from build123d import *

# Parameters (mm, degrees)
ESBO_O1_W                = 111
ESBO_O1_H                = 40
RESSALTO_EXTRUS_O1_DEPTH = 18
ESBO_O2_W                = 2
ESBO_O2_H                = 16
ESBO_O2_H_2              = 21
ESBO_O2_H_3              = 40
RESSALTO_EXTRUS_O2_DEPTH = 13
RESSALTO_EXTRUS_O3_REACH = 68.643
ESBO_O3_W                = 3
ESBO_O3_H                = 7.5
ESBO_O4_R                = 1.65
CORTE_EXTRUS_O1_DEPTH    = 6
FILETE1_R                = 5


with BuildPart() as part:
    # Esboço1 → Ressalto-extrusão1 (new body)
    with BuildSketch(Plane.XY):
        Rectangle(ESBO_O1_W, ESBO_O1_H)
    extrude(amount=RESSALTO_EXTRUS_O1_DEPTH)

    # Esboço2 → Ressalto-extrusão2 (add)
    with BuildSketch(Plane.XY.offset(18)):
        with Locations((-28.2, -12)):
            Rectangle(ESBO_O2_W, ESBO_O2_H)
        with Locations((-23.072727273, -12)):
            Rectangle(ESBO_O2_W, ESBO_O2_H)
        with Locations((-17.945454545, -12)):
            Rectangle(ESBO_O2_W, ESBO_O2_H)
        with Locations((-12.818181818, -12)):
            Rectangle(ESBO_O2_W, ESBO_O2_H)
        with Locations((-7.690909091, -12)):
            Rectangle(ESBO_O2_W, ESBO_O2_H)
        with Locations((-2.563636364, -12)):
            Rectangle(ESBO_O2_W, ESBO_O2_H)
        with Locations((2.563636364, -12)):
            Rectangle(ESBO_O2_W, ESBO_O2_H)
        with Locations((7.690909091, -12)):
            Rectangle(ESBO_O2_W, ESBO_O2_H)
        with Locations((12.818181818, -12)):
            Rectangle(ESBO_O2_W, ESBO_O2_H)
        with Locations((17.945454545, -12)):
            Rectangle(ESBO_O2_W, ESBO_O2_H)
        with Locations((23.072727273, -12)):
            Rectangle(ESBO_O2_W, ESBO_O2_H)
        with Locations((28.2, -12)):
            Rectangle(ESBO_O2_W, ESBO_O2_H)
        with Locations((-47.9, 0)):
            Rectangle(ESBO_O2_W, ESBO_O2_H_2)
        with Locations((-52.9, 0)):
            Rectangle(ESBO_O2_W, ESBO_O2_H_2)
        with Locations((-42.9, 0)):
            Rectangle(ESBO_O2_W, ESBO_O2_H_3)
        with Locations((-37.9, 0)):
            Rectangle(ESBO_O2_W, ESBO_O2_H_3)
        with Locations((-32.9, 0)):
            Rectangle(ESBO_O2_W, ESBO_O2_H_3)
        with Locations((32.9, 0)):
            Rectangle(ESBO_O2_W, ESBO_O2_H_3)
        with Locations((37.9, 0)):
            Rectangle(ESBO_O2_W, ESBO_O2_H_3)
        with Locations((42.9, 0)):
            Rectangle(ESBO_O2_W, ESBO_O2_H_3)
        with Locations((47.9, 0)):
            Rectangle(ESBO_O2_W, ESBO_O2_H_2)
        with Locations((52.9, 0)):
            Rectangle(ESBO_O2_W, ESBO_O2_H_2)
    extrude(amount=RESSALTO_EXTRUS_O2_DEPTH)

    # Esboço3 → Ressalto-extrusão3 (add, up to next)
    with BuildSketch(Plane.XY.offset(31), mode=Mode.PRIVATE) as ressalto_extrus_o3_sk1:
        with Locations((-40.4, -11.95)):
            Rectangle(ESBO_O3_W, ESBO_O3_H)
    ressalto_extrus_o3_tool1 = extrude(ressalto_extrus_o3_sk1.sketch, amount=-RESSALTO_EXTRUS_O3_REACH, mode=Mode.PRIVATE) - part.part
    # Esboço3 → Ressalto-extrusão3 (add, up to next)
    with BuildSketch(Plane.XY.offset(31), mode=Mode.PRIVATE) as ressalto_extrus_o3_sk2:
        with Locations((-35.4, -11.95)):
            Rectangle(ESBO_O3_W, ESBO_O3_H)
    ressalto_extrus_o3_tool2 = extrude(ressalto_extrus_o3_sk2.sketch, amount=-RESSALTO_EXTRUS_O3_REACH, mode=Mode.PRIVATE) - part.part
    # Esboço3 → Ressalto-extrusão3 (add, up to next)
    with BuildSketch(Plane.XY.offset(31), mode=Mode.PRIVATE) as ressalto_extrus_o3_sk3:
        with Locations((35.4, -11.95)):
            Rectangle(ESBO_O3_W, ESBO_O3_H)
    ressalto_extrus_o3_tool3 = extrude(ressalto_extrus_o3_sk3.sketch, amount=-RESSALTO_EXTRUS_O3_REACH, mode=Mode.PRIVATE) - part.part
    # Esboço3 → Ressalto-extrusão3 (add, up to next)
    with BuildSketch(Plane.XY.offset(31), mode=Mode.PRIVATE) as ressalto_extrus_o3_sk4:
        with Locations((40.4, -11.95)):
            Rectangle(ESBO_O3_W, ESBO_O3_H)
    ressalto_extrus_o3_tool4 = extrude(ressalto_extrus_o3_sk4.sketch, amount=-RESSALTO_EXTRUS_O3_REACH, mode=Mode.PRIVATE) - part.part
    add(ressalto_extrus_o3_tool1.solids().sort_by_distance((-40.4, -11.95, 31))[0])
    add(ressalto_extrus_o3_tool2.solids().sort_by_distance((-35.4, -11.95, 31))[0])
    add(ressalto_extrus_o3_tool3.solids().sort_by_distance((35.4, -11.95, 31))[0])
    add(ressalto_extrus_o3_tool4.solids().sort_by_distance((40.4, -11.95, 31))[0])

    # Esboço4 → Corte-extrusão1 (cut)
    with BuildSketch(Plane.XY.offset(31)):
        with Locations((-37.9, -11.95)):
            Circle(ESBO_O4_R)
        with Locations(Location((37.9, -11.95, 0), (0, 0, 180))):
            Circle(ESBO_O4_R)
    extrude(amount=-CORTE_EXTRUS_O1_DEPTH, mode=Mode.SUBTRACT)

    # Filete1
    filete1_edges = [part.edges().sort_by_distance(p)[0] for p in [
        (-55.5, 20, 9),
        (55.5, 20, 9),
        (55.5, -20, 9),
        (-55.5, -20, 9),
    ]]
    fillet(filete1_edges, radius=FILETE1_R)


solid = part.part
The model under review builds one solid part; all positions refer to its coordinate system, in mm. A direction names the side the tool comes from. Give positions to 0.01 mm unless a question says otherwise; leave off trailing zeros. Order: outer loops, then holes, each group sorted by start corner. A loop starts at its lowest first (then second) coordinate and runs counter-clockwise, first axis right, second up. Notation, with made-up numbers: M 17,-35 L 53,-35 A14 ccw 53,-9 Z; hole C 10,67 d2. An arc over 180 degrees is marked long. Answer in a Markdown table with one row per item. Add a question column.
1. Mouldability with a two-part tool opening along X and no side actions: class faces 1 (the flat face through (-8, -12, 31)), 2 (the flat face through (-40, -8.2, 25)), 3 (the cylindrical face through (-54.07, 18.5, 9.13)) as released by +X, released by -X, zero draft, split by the parting line, or undercut.
2. For pin 1 Ø1.5 at (x, y) = (-41, -18) entering from +Z; pin 2 Ø1 at (x, z) = (7, 26.5) entering from +Y; pin 3 Ø0.6 at (x, z) = (-48, 27.5) entering from +Y, all flat-tipped, find the tip position at first contact; note any pin that passes through.
3. To check wall thickness, follow line 1 along Y through (x, z) = (-37.9, 27.3); line 2 along Z through (x, y) = (8.5, 11); line 3 along Y through (x, z) = (41, 24.5). State the ranges of each line that lie inside material, in increasing order.
4. Add section A-A on x = -37.9. State the section outline as (y, z) points.
5. Add section C-C on x = 20. State the section outline as (y, z) points, plus the area to 3 significant figures.
6. Add section B-B on z = 26.5. Count the separate pieces of the cut face and the enclosed holes in it, plus the area to 3 significant figures.
7. Machinability: for faces 4 (the flat face through (-28, -4, 24)), 5 (the flat face through (-41.9, -18, 24)), 6 (the flat face through (-48, 10.5, 24)), 7 (the flat face through (24.073, -12, 24)), which of the approach directions +Z, -Z, +X, -X, +Y, -Y give a long, thin tool a straight path to every point of the face, cutting with its end or side? Answer none if there is none.
The answers:
| question | item | result |
|---|---|---|
| 1 | face 1 | zero draft |
| 1 | face 2 | undercut |
| 1 | face 3 | released by -X |
| 2 | pin 1 | z = 18 |
| 2 | pin 2 | y = -4 |
| 2 | pin 3 | y = 10.5 |
| 3 | line 1 | -20 to -13.6, -10.3 to 20 |
| 3 | line 2 | 0 to 18 |
| 3 | line 3 | -15.7 to -8.2 |
| 4 | outline | M -20,0 L 20,0 L 20,31 L -10.3,31 L -10.3,25 L -13.6,25 L -13.6,31 L -20,31 Z |
| 5 | outline | M -20,0 L 20,0 L 20,18 L -20,18 Z |
| 5 | area | 720 mm2 |
| 6 | separate pieces | 18 |
| 6 | enclosed holes | 2 |
| 6 | area | 1,100 mm2 |
| 7 | face 4 | +Z, +Y |
| 7 | face 5 | +Z, -Y |
| 7 | face 6 | +Z, -X, +Y |
| 7 | face 7 | +Z, +Y, -Y |
